```python
from build123d import *

# Parameters (mm, degrees)
F1_DEPTH = 152.4
F2_START = 25.4
F0_W     = 520.7
F0_H     = 1098.55
F2_DEPTH = 9.525
F3_W     = 95.25
F3_H     = 254
F4_DEPTH = 45.72


with BuildPart() as f1:
    # F0 (on Front) → F1 (new body)
    with BuildSketch(Plane.XZ):
        Polygon((259.2205437755, 656.2005733788), (-299.5794562245, 656.2005733788), (-299.5794562245, -461.3994266212), (-280.5294562245, -461.3994266212), (-280.5294562245, 637.1505733788), (240.1705437755, 637.1505733788), (240.1705437755, -461.3994266212), (259.2205437755, -461.3994266212), align=None)
    extrude(amount=F1_DEPTH)

    # F0 (on Front) → F2 (join)
    with BuildSketch(Plane.XZ.offset(F2_START)):
        with Locations((-20.1794562245, 87.8755733788)):
            Rectangle(F0_W, F0_H)
    extrude(amount=F2_DEPTH)

    # F3 (on face) → F4 (join)
    with BuildSketch(Plane.XZ.offset(34.925)):
        with Locations((-170.6612408161, 391.3649345023)):
            Rectangle(F3_W, F3_H)
    extrude(amount=F4_DEPTH)


solid = f1.part
```
Geometry check sheet. Reference: the model listing, model coordinates, mm. A direction names the side the tool comes from. Coordinates: 2 decimals unless noted, no trailing zeros. Loops run counter-clockwise (first coordinate to the right, second up) from the corner with the lowest first, then second, coordinate; pieces in that order, holes last.
Item 1: Sectioned sample at A-A, the plane y = -69. Record the boundary of the cut face in (x, z).
Item 2: Sectioned sample at C-C, the plane z = 410. Record the boundary of the cut face in (x, y) (3 decimals), then the cut area to 3 significant figures.
Item 3: Release check for a two-part mould opening along X. For faces 1 (the face through (-171, -57, 264.365)), 2 (the face through (259.221, -75, 90)), 3 (the face through (-291, -152.4, 266)), 4 (the face through (-171, -80.645, 393)) record: released by +X, released by -X, zero draft, split by the parting line, or undercut.
Item 4: Sectioned sample at B-B, the plane x = 37.5. Record the boundary of the cut face in (y, z) (3 decimals), then the cut area to 3 significant figures.
Item 5: Thickness scan on line 1 (X direction, y = -61.5, z = 444.5); line 2 (X direction, y = -79.5, z = 144.5); line 3 (Z direction, x = -189, y = -103.5). Record the ranges inside material, lowest first.
Item 6: Go/stop test with flat-tipped pins: pin 1 Ø3 at (x, z) = (111, -24.5) entering from +Y; pin 2 Ø3 at (x, y) = (-163.5, -101.5) entering from -Z; pin 3 Ø6 at (x, z) = (-235.5, 431) entering from -Y (3 decimals). Record where each tip stops, or that it passes through.
Item 7: Sectioned sample at D-D, the plane y = -129.5. Record the boundary of the cut face in (x, z), then the cut area to 3 significant figures.
Item 8: Access from +Z, -Z, +X, -X, +Y, -Y to the whole of each face (thin tool, end or side, straight path). Record for faces 5 (the face through (-280.529, -93, 80)), 6 (the face through (-171, -57, 518.365)), 7 (the face through (-280.529, -13, 80)).
Check result:
1. outline: (-299.58, -461.4) - (-280.53, -461.4) - (-280.53, 637.15) - (240.17, 637.15) - (240.17, -461.4) - (259.22, -461.4) - (259.22, 656.2) - (-299.58, 656.2) - close; (-218.29, 264.36) - (-123.04, 264.36) - (-123.04, 518.36) - (-218.29, 518.36) - close
2. outline: (-299.579, -152.4) - (-280.529, -152.4) - (-280.529, -34.925) - (-218.286, -34.925) - (-218.286, -80.645) - (-123.036, -80.645) - (-123.036, -34.925) - (240.171, -34.925) - (240.171, -152.4) - (259.221, -152.4) - (259.221, 0) - (240.171, 0) - (240.171, -25.4) - (-280.529, -25.4) - (-280.529, 0) - (-299.579, 0) - close
2. area: 15,100 mm2
3. face 1: undercut
3. face 2: released by +X
3. face 3: zero draft
3. face 4: undercut
4. outline: (-152.4, 637.151) - (-34.925, 637.151) - (-34.925, -461.399) - (-25.4, -461.399) - (-25.4, 637.151) - (0, 637.151) - (0, 656.201) - (-152.4, 656.201) - close
4. area: 13,400 mm2
5. line 1: x = -299.58 to -280.53, -218.29 to -123.04, 240.17 to 259.22
5. line 2: x = -299.58 to -280.53, 240.17 to 259.22
5. line 3: z = 637.15 to 656.2
6. pin 1: stops at y = -25.4
6. pin 2: stops at z = 637.15
6. pin 3: stops at y = -34.925
7. outline: (-299.58, -461.4) - (-280.53, -461.4) - (-280.53, 637.15) - (240.17, 637.15) - (240.17, -461.4) - (259.22, -461.4) - (259.22, 656.2) - (-299.58, 656.2) - close
7. area: 52,500 mm2
8. face 5: -Z, -Y
8. face 6: -Y
8. face 7: -Z, +Y
